Part print with two shaded views. Sizes in mm from the minimum x, y, z corner. A direction names the side the tool comes from. Round coordinates to 2 decimals unless told otherwise and drop trailing zeros. Write each loop counter-clockwise with the first axis right and the second up, starting at its lowest first coordinate (ties: lowest second). Pieces come first, ordered by that corner, then holes. Notation, with made-up numbers: M -12,87 L 11,87 A15 cw 11,97 Z; hole C -3,9 d2. An arc over 180 degrees is marked long. One line per question, with ' | ' between items. Start each with the question number.
1) Saw through at B-B (z = 2.75). List the corners of the cut face in (x, y).
2) Saw through at A-A (x = 25.5). List the corners of the cut face in (y, z).
3) Tool access for the marked faces 1, 2, 3 and 4: list every direction of +Z, -Z, +X, -X, +Y, -Y with a clear straight run to the whole face (end or side of a thin tool).
4) Saw through at C-C (y = 2). List the corners of the cut face in (x, z), plus the area to 3 significant figures.
5) Drop flat-ended pins along their axis: pin 1 Ø1 at (x, y) = (32.3, 9.375) entering from +Z; pin 2 Ø1 at (y, z) = (5, 1) entering from +X; pin 3 Ø2 at (x, z) = (31.5, 1) entering from +Y; pin 4 Ø2 at (x, z) = (3, 1) entering from -Y. Give the stop position or say it passes through.
6) Wall check: probe 1 along Y at (x, z) = (2, 0.8) (1 decimal); probe 2 along X at (y, z) = (8.5, 6); probe 3 along Y at (x, z) = (11, 2.75). Give the ranges that are in metal, low to high. Write a range as [from, to].
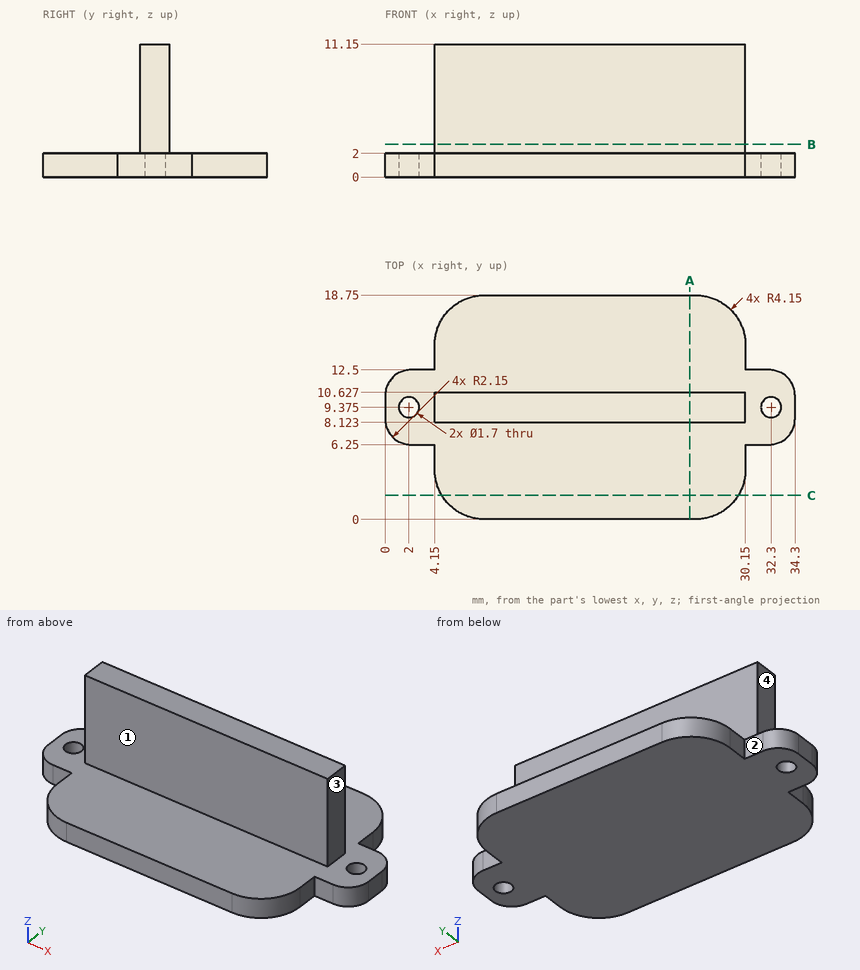
Answer key:
1) outline: M 4.15,8.12 L 30.15,8.12 L 30.15,10.63 L 4.15,10.63 Z
2) outline: M 0,0 L 18.75,0 L 18.75,2 L 10.63,2 L 10.63,11.15 L 8.12,11.15 L 8.12,2 L 0,2 Z
3) face 1: +Z, +X, -X, -Y | face 2: +Z, -Z, -X, +Y | face 3: +Z, +X, +Y, -Y | face 4: +Z, -X, +Y, -Y
4) outline: M 4.75,0 L 29.55,0 L 29.55,2 L 4.75,2 Z | area: 49.6 mm2
5) pin 1: passes through | pin 2: stops at x = 30.15 | pin 3: stops at y = 12.5 | pin 4: stops at y = 6.25
6) probe 1: y = [6.3, 8.5], [10.2, 12.5] | probe 2: x = [4.15, 30.15] | probe 3: y = [8.12, 10.63]
